from build123d import *

# Parameters (mm, degrees)
BOSS_EXTRUDE1_DEPTH      = 5.08
BOSS_EXTRUDE1_DEPTH_BACK = 5.08
SKETCH2_R                = 0.79375
SKETCH3_R                = 1.4986
BOSS_EXTRUDE3_DEPTH      = 4.9276


with BuildPart() as part:
    # Sketch1 → Revolve1 (revolve)
    with BuildSketch(Plane.XY):
        with BuildLine():
            Line((0, 0), (0, 22.572427826))
            Line((0, 22.572427826), (4.37022875, 22.572427826))
            Line((4.37022875, 22.572427826), (4.54025, 24.858427826))
            Line((4.54025, 24.858427826), (5.30225, 24.858427826))
            Line((5.30225, 24.858427826), (4.5466, 14.698427826))
            Line((4.5466, 14.698427826), (4.5466, 3.522427826))
            Line((4.5466, 3.522427826), (2.86385, 3.522427826))
            Line((2.86385, 3.522427826), (1.778, 1.143))
            ThreePointArc((1.778, 1.143), (1.056850628, 0.310399023), (0, 0))
        make_face()
    revolve(axis=Axis((0, 0, 0), (0, 1, 0)))

    # Sketch2 → Boss-Extrude1 (add, two sides: drawn at the far end of the back side and taken through both)
    with BuildSketch(Plane(origin=(0, 0, 0), x_dir=(0, 0, -1), z_dir=(1, 0, 0)).offset(-BOSS_EXTRUDE1_DEPTH_BACK)):
        with Locations((0, 4.646377826)):
            Circle(SKETCH2_R)
    extrude(amount=BOSS_EXTRUDE1_DEPTH + BOSS_EXTRUDE1_DEPTH_BACK)

    # Sketch3 → Boss-Extrude3 (add)
    with BuildSketch(Plane(origin=(0, 22.572427826, 0), x_dir=(1, 0, 0), z_dir=(0, 1, 0))):
        with Locations(Location((-1.92644128, 0.516188385, 0), (0, 0, 270))):
            Circle(SKETCH3_R)
        with Locations(Location((1.410252895, 1.410252895, 0), (0, 0, 270))):
            Circle(SKETCH3_R)
        with Locations(Location((0.516188385, -1.92644128, 0), (0, 0, 270))):
            Circle(SKETCH3_R)
    extrude(amount=BOSS_EXTRUDE3_DEPTH)


solid = part.part
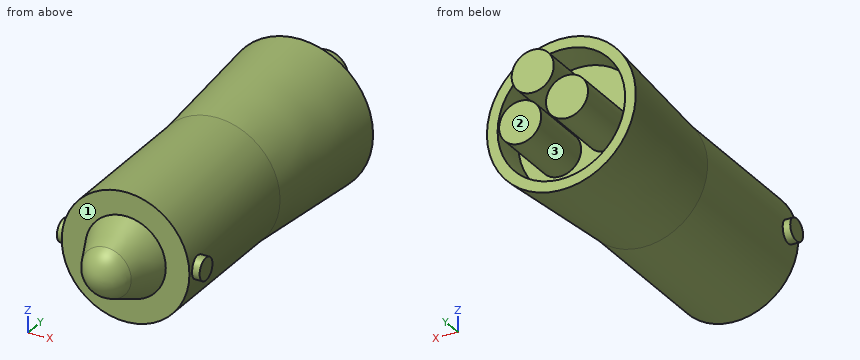
Can you work these out from the model? Positions are in its coordinate system, mm. Face numbers are marked on the shaded views. A direction names the side the tool comes from. Round coordinates to 2 decimals unless told otherwise and drop trailing zeros. Order: outer loops, then holes, each group sorted by start corner. A loop starts at its lowest first (then second) coordinate and runs counter-clockwise, first axis right, second up. Notation, with made-up numbers: (72.5, -37.5) -> (91.5, -37.5) arc R15 ccw to (91.5, -31.5) -> close; hole circle Ø8 at (82, 3.25). An arc over 180 degrees is marked (long way). Write each question's results on one line, items separated by ' | '. Start each with the question number.
Item 1: If we section it at A-A, the plane y = 23.75: Write out the boundary of the cut face in (x, z), then the cut area to 3 significant figures.
Item 2: If we section it at B-B, the plane y = 10: Write out the boundary of the cut face in (x, z).
Item 3: Please list where these lines run through material, in increasing order: L1, parallel to X at y = 23.5, z = -2.25; L2, parallel to Y at x = -2.25, z = 2; L3, parallel to X at y = 26.25, z = -1.25.
Item 4: Which directions (+Z, -Z, +X, -X, +Y, -Y) give clear straight access to the entire face, cutting with the end or side of a thin tool? Please do the marked faces 1, 2 and 3.
Item 5: Will these pins go through, and if not, where does the flat tip stop? pin 1 (1.5 mm diameter, centred on x = 2, y = 5, fed in from -Z); pin 2 (3 mm diameter, centred on x = -2.5, y = 20, fed in from +Z); pin 3 (6 mm diameter, centred on y = 6.5, z = -2, fed in from -X).
Item 6: If we section it at D-D, the plane y = 15.75: Write out the boundary of the cut face in (x, z).
Results:
1) outline: circle Ø10.44 at (0, 0); circle Ø3 at (-1.93, -0.52); circle Ø3 at (0.52, 1.93); circle Ø3 at (1.41, -1.41); hole circle Ø8.92 at (0, 0) | area: 44.3 mm2
2) outline: circle Ø9.09 at (0, 0)
3) L1: x = -4.69 to -3.83, 0.17 to 2.65, 3.83 to 4.69 | L2: y = 3.52 to 22.57 | L3: x = -3.23 to -0.62, -0.08 to 2.9
4) face 1: -Y | face 2: +Z, -Z, +X, -X, +Y | face 3: +Y
5) pin 1: stops at z = -4.37 | pin 2: stops at z = 4.86 | pin 3: stops at x = -5.08
6) outline: circle Ø9.25 at (0, 0)
